```python
from build123d import *
from build123d.topology import SkipClean

# Parameters (mm, degrees)
BOSS_EXTRUDE1_DEPTH     = 17
SKETCH3_R               = 1.5
CUT_EXTRUDE1_DEPTH      = 27.365887051
SKETCH4_3_R             = 1.5
CUT_EXTRUDE3_DEPTH      = 1.8
CUT_EXTRUDE2_DEPTH      = 26.439339614
CUT_EXTRUDE2_DEPTH_BACK = 26.439339614
SKETCH4_R               = 1.5
SKETCH3_3_R             = 1.5
CUT_EXTRUDE4_DEPTH      = 1.45
SKETCH6_W               = 5.542562584
SKETCH6_H               = 1.8
CUT_EXTRUDE5_DEPTH      = 3.2
SKETCH7_W               = 2.771281292
SKETCH7_H               = 1.8
CUT_EXTRUDE6_DEPTH      = 24.538054295


with BuildPart() as part:
    # Sketch2 → Boss-Extrude1 (new body)
    with BuildSketch(Plane.XY):
        Polygon((0, 0), (6.875, 0), (6.875, 10), (8.525, 10), (8.525, 0), (15.4, 0), (15.4, 13), (0, 13), align=None)
    extrude(amount=-BOSS_EXTRUDE1_DEPTH)

    # Sketch3 → Cut-Extrude1 (cut, through all)
    with BuildSketch(Plane(origin=(15.4, 0, 0), x_dir=(0, 0, -1), z_dir=(1, 0, 0))):
        with Locations(Location((11.71, 4.99, 0), (0, 0, 90))):
            Circle(SKETCH3_R)
    extrude(amount=-CUT_EXTRUDE1_DEPTH, mode=Mode.SUBTRACT)

    # Sketch4<3> → Cut-Extrude3 (cut)
    # profile 1 of 4: a face of its own
    with BuildSketch(Plane(origin=(0, 11, 0), x_dir=(1, 0, 0), z_dir=(0, 1, 0))):
        with Locations(Location((3.2, 4.5, 0), (0, 0, 180))):
            Circle(SKETCH4_3_R)
    # profile 2 of 4: a face of its own
    with BuildSketch(Plane(origin=(0, 11, 0), x_dir=(1, 0, 0), z_dir=(0, 1, 0))):
        with Locations((12.2, 4.5)):
            Circle(SKETCH4_3_R)
    # profile 3 of 4: a face of its own
    with BuildSketch(Plane(origin=(0, 11, 0), x_dir=(1, 0, 0), z_dir=(0, 1, 0))):
        Polygon((9.8, 12.114359354), (9.8, 14.885640646), (12.2, 16.271281292), (14.6, 14.885640646), (14.6, 12.114359354), (12.2, 10.728718708), align=None)
        with Locations((12.2, 13.5)):
            Circle(SKETCH4_3_R, mode=Mode.SUBTRACT)
    # profile 4 of 4: a face of its own
    with BuildSketch(Plane(origin=(0, 11, 0), x_dir=(1, 0, 0), z_dir=(0, 1, 0))):
        Polygon((3.2, 16.271281292), (0.8, 14.885640646), (0.8, 12.114359354), (3.2, 10.728718708), (5.6, 12.114359354), (5.6, 14.885640646), align=None)
        with Locations(Location((3.2, 13.5, 0), (0, 0, 180))):
            Circle(SKETCH4_3_R, mode=Mode.SUBTRACT)
    extrude(amount=-CUT_EXTRUDE3_DEPTH, mode=Mode.SUBTRACT)

    # Sketch4 → Cut-Extrude2 (cut, two sides: drawn at the far end of the back side and taken through both)
    with SkipClean():  # the faces are left unmerged after this step: merging them gives an invalid solid
        with BuildSketch(Plane(origin=(0, 11, 0), x_dir=(1, 0, 0), z_dir=(0, 1, 0)).offset(-CUT_EXTRUDE2_DEPTH_BACK)):
            with Locations(Location((3.2, 13.5, 0), (0, 0, 180))):
                Circle(SKETCH4_R)
            with Locations(Location((12.2, 13.5, 0), (0, 0, 180))):
                Circle(SKETCH4_R)
            with Locations(Location((3.2, 4.5, 0), (0, 0, 180))):
                Circle(SKETCH4_R)
            with Locations(Location((12.2, 4.5, 0), (0, 0, 180))):
                Circle(SKETCH4_R)
        extrude(amount=CUT_EXTRUDE2_DEPTH + CUT_EXTRUDE2_DEPTH_BACK, mode=Mode.SUBTRACT)

    # Sketch3<3> → Cut-Extrude4 (cut)
    with SkipClean():  # the faces are left unmerged after this step: merging them gives an invalid solid
        with BuildSketch(Plane(origin=(15.4, 0, 0), x_dir=(0, 0, -1), z_dir=(1, 0, 0))):
            Polygon((14.065, 3.630340116), (11.71, 2.270680232), (9.355, 3.630340116), (9.355, 6.349659884), (11.71, 7.709319768), (14.065, 6.349659884), align=None)
            with Locations(Location((11.71, 4.99, 0), (0, 0, 90))):
                Circle(SKETCH3_3_R, mode=Mode.SUBTRACT)
        cut_extrude4 = extrude(amount=-CUT_EXTRUDE4_DEPTH, mode=Mode.SUBTRACT)

    # Mirror1: Cut-Extrude4 across plane
    with SkipClean():  # the faces are left unmerged after this step: merging them gives an invalid solid
        add(cut_extrude4.mirror(Plane(origin=(7.7, 0, 0), x_dir=(0, 0, 1), z_dir=(1, 0, 0))), mode=Mode.SUBTRACT)

    # Sketch6 → Cut-Extrude5 (cut)
    with SkipClean():  # the faces are left unmerged after this step: merging them gives an invalid solid
        with BuildSketch(Plane.ZY):
            with Locations((-13.5, 10.1)):
                Rectangle(SKETCH6_W, SKETCH6_H)
        cut_extrude5 = extrude(amount=-CUT_EXTRUDE5_DEPTH, mode=Mode.SUBTRACT)

    # Sketch7 → Cut-Extrude6 (cut, through all)
    with SkipClean():  # the faces are left unmerged after this step: merging them gives an invalid solid
        with BuildSketch(Plane.ZY.offset(-5.6)):
            with Locations((-13.5, 10.1)):
                Rectangle(SKETCH7_W, SKETCH7_H)
        extrude(amount=-CUT_EXTRUDE6_DEPTH, mode=Mode.SUBTRACT)

    # Mirror2: Cut-Extrude5 across plane
    with SkipClean():  # the faces are left unmerged after this step: merging them gives an invalid solid
        add(cut_extrude5.mirror(Plane(origin=(7.7, 0, 0), x_dir=(0, 0, 1), z_dir=(1, 0, 0))), mode=Mode.SUBTRACT)


solid = part.part
```
Work out the finished part from the listing and answer in its coordinate system (mm). A direction names the side the tool comes from. Give positions to 0.01 mm unless a question says otherwise; leave off trailing zeros. Order: outer loops, then holes, each group sorted by start corner. A loop starts at its lowest first (then second) coordinate and runs counter-clockwise, first axis right, second up. Notation, with made-up numbers: M 78,-1.75 L 85,-1.75 A14 cw 85,19.25 Z; hole C -17.5,55 d11. An arc over 180 degrees is marked long. Return JSON: item names as keys, results as strings.
1) Each of these flat-tipped pins is pushed along its axis until it touches: pin 1 (4 mm diameter, centred on x = 12.2, z = -13.5, fed in from +Y); pin 2 (2.5 mm diameter, centred on y = 6, z = -12, fed in from -X); pin 3 (1 mm diameter, centred on x = 7.5, z = -8.5, fed in from -Y). Where does it stop, or does it pass through?
Resolved:
{"pin 1": "y = 13", "pin 2": "x = 1.45", "pin 3": "y = 10"}
2) Straight lines are drawn through the part: line 1 along X through (y, z) = (3, -13.5) (3 decimals); line 2 along X through (y, z) = (12.1, -13.5); line 3 along X through (y, z) = (9.5, -2.5) (3 decimals). For each, find the intervals that lie inside material, in ascending order. Write a range as [from, to].
Resolved:
{"line 1": "[0, 1.7], [4.7, 6.875], [8.525, 10.7], [13.7, 15.4]", "line 2": "[0, 1.7], [4.7, 10.7], [13.7, 15.4]", "line 3": "[0, 6.875], [8.525, 15.4]"}
3) For a pull along X with two mould halves and no side action, classify faces 5 (the flat face through (11.02, 10.11, -11.41)), 6 (the flat face through (6, 7, -17)), 7 (the cylindrical face through (10.814, 11.986, -14.075)) as +X half, -X half, draft (parallel to the pull), parting line (faces both ways), or undercut.
Resolved:
{"face 5": "+X half", "face 6": "draft", "face 7": "undercut"}
4) Section A-A, the plane y = 1.75 is taken. Write down the section's boundary in (x, z) (3 decimals).
Resolved:
{"outline": "M 0,-17 L 6.875,-17 L 6.875,0 L 0,0 Z; M 8.525,-17 L 15.4,-17 L 15.4,0 L 8.525,0 Z; hole C 3.2,-13.5 d3; hole C 3.2,-4.5 d3; hole C 12.2,-13.5 d3; hole C 12.2,-4.5 d3"}
5) Section D-D, the plane x = 9 is taken. Write down the section's boundary in (y, z).
Resolved:
{"outline": "M 0,-17 L 13,-17 L 13,0 L 0,0 Z; hole C 4.99,-11.71 d3; hole M 9.2,-14.89 L 11,-14.89 L 11,-12.11 L 9.2,-12.11 Z"}
6) Section C-C, the plane y = 10.75 is taken. Write down the section's boundary in (x, z), plus the area to 3 significant figures.
Resolved:
{"outline": "M 0,-17 L 15.4,-17 L 15.4,-16.27 L 12.2,-16.27 L 9.8,-14.89 L 5.6,-14.89 L 3.2,-16.27 L 0,-16.27 Z; M 0,-10.73 L 3.2,-10.73 L 5.6,-12.11 L 9.8,-12.11 L 12.2,-10.73 L 15.4,-10.73 L 15.4,0 L 0,0 Z; hole C 3.2,-4.5 d3; hole C 12.2,-4.5 d3", "area": "181 mm^2"}
7) Section B-B, the plane z = -4.5 is taken. Write down the section's boundary in (x, y) (3 decimals).
Resolved:
{"outline": "M 0,0 L 1.7,0 L 1.7,13 L 0,13 Z; M 4.7,0 L 6.875,0 L 6.875,10 L 8.525,10 L 8.525,0 L 10.7,0 L 10.7,13 L 4.7,13 Z; M 13.7,0 L 15.4,0 L 15.4,13 L 13.7,13 Z"}
8) A tool of negligible diameter and unlimited length cuts with its end or side. For faces 1 (the flat face through (14, 10, -10.729)), 2 (the cylindrical face through (12.525, 4.536, -14.964)), 3 (the flat face through (7.7, 10.3, -14.886)), 4 (the flat face through (4.417, 10.113, -15.569)), from which of +Z, -Z, +X, -X, +Y, -Y can it reach the whole face along a straight path? Write none if from no direction.
Resolved:
{"face 1": "+X", "face 2": "+Y, -Y", "face 3": "+X, -X", "face 4": "-X"}
